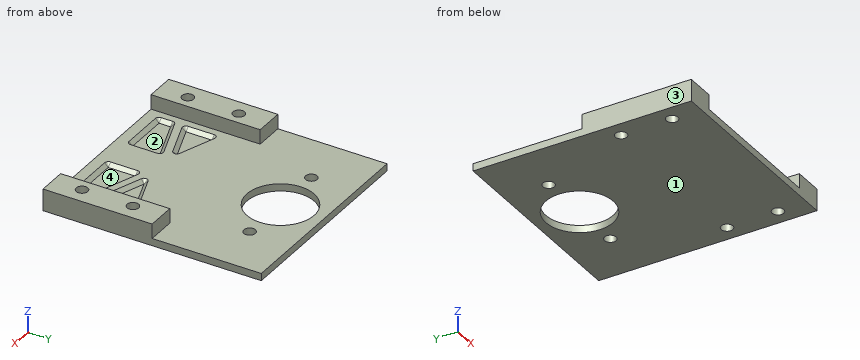
from build123d import *

# Parameters (mm, degrees)
SKIZZE1_W                       = 57
SKIZZE1_H                       = 60
GRUNDPLATTE_DEPTH               = 2
SKIZZE2_R                       = 9.25
SKIZZE2_R_2                     = 1.6
AUSSCHNITT_ROLLE_DEPTH          = 67.454871906
SKIZZE4_W                       = 8
SKIZZE4_H                       = 30
AUFSATZ_GETRIEBE_DEPTH          = 4
BOHRUNGEN_START                 = 4
SKIZZE3_R                       = 1.6
BOHRUNGEN_GETRIEBE_DEPTH        = 71.54509749
SCHNITT_LINEAR_AUSTRAGEN3_DEPTH = 1
VERRUNDUNG1_R                   = 1
FASE1_SIZE                      = 1


with BuildPart() as part:
    # Skizze1 → Grundplatte (new body)
    with BuildSketch(Plane.XY):
        with Locations((0, 30)):
            Rectangle(SKIZZE1_W, SKIZZE1_H)
    extrude(amount=GRUNDPLATTE_DEPTH)

    # Skizze2 → Ausschnitt_Rolle (cut, through all)
    with BuildSketch(Plane.XY.offset(2)):
        with Locations((0, 48)):
            Circle(SKIZZE2_R)
        with Locations((-14, 48)):
            Circle(SKIZZE2_R_2)
        with Locations(Location((14, 48, 0), (0, 0, 180))):
            Circle(SKIZZE2_R_2)
    extrude(amount=-AUSSCHNITT_ROLLE_DEPTH, mode=Mode.SUBTRACT)

    # Skizze4 → Aufsatz Getriebe (add)
    with BuildSketch(Plane.XY.offset(2)):
        with Locations((24.5, 15)):
            Rectangle(SKIZZE4_W, SKIZZE4_H)
        with Locations((-24.5, 15)):
            Rectangle(SKIZZE4_W, SKIZZE4_H)
    extrude(amount=AUFSATZ_GETRIEBE_DEPTH)

    # Skizze3 → Bohrungen Getriebe (cut, through all)
    with BuildSketch(Plane.XY.offset(2).offset(BOHRUNGEN_START)):
        with Locations(Location((-24, 22, 0), (0, 0, 180))):
            Circle(SKIZZE3_R)
        with Locations(Location((-24, 8, 0), (0, 0, 180))):
            Circle(SKIZZE3_R)
        with Locations(Location((24, 8, 0), (0, 0, 180))):
            Circle(SKIZZE3_R)
        with Locations(Location((24, 22, 0), (0, 0, 180))):
            Circle(SKIZZE3_R)
    extrude(amount=-BOHRUNGEN_GETRIEBE_DEPTH, mode=Mode.SUBTRACT)

    # Skizze5 → Schnitt-Linear austragen3 (cut)
    with BuildSketch(Plane.XY.offset(2)):
        Polygon((-18.5, 20), (-18.5, 10), (-4.5, 15), align=None)
        Polygon((-18.5, 7.876275893), (-18.5, 3), (-4.5, 3), (-4.5, 12.876275893), align=None)
        Polygon((4.5, 12.876275893), (18.5, 7.876275893), (18.5, 3), (4.5, 3), align=None)
        Polygon((4.5, 15), (18.5, 20), (18.5, 10), align=None)
    extrude(amount=-SCHNITT_LINEAR_AUSTRAGEN3_DEPTH, mode=Mode.SUBTRACT)

    # Verrundung1
    verrundung1_edges = [part.edges().sort_by_distance(p)[0] for p in [
        (-18.5, 3, 1.5),
        (-4.5, 3, 1.5),
        (-4.5, 12.876275893, 1.5),
        (-18.5, 7.876275893, 1.5),
        (18.5, 20, 1.5),
        (4.5, 15, 1.5),
        (18.5, 10, 1.5),
        (18.5, 3, 1.5),
        (18.5, 7.876275893, 1.5),
        (4.5, 12.876275893, 1.5),
        (4.5, 3, 1.5),
        (-18.5, 10, 1.5),
        (-4.5, 15, 1.5),
        (-18.5, 20, 1.5),
    ]]
    fillet(verrundung1_edges, radius=VERRUNDUNG1_R)

    # Fase1
    fase1_edges = [part.edges().sort_by_distance(p)[0] for p in [
        (4.923951563, 12.274686543, 1),
        (11.836336397, 10.256155751, 1),
        (18.31741556, 7.747605134, 1),
        (18.5, 5.585778349, 1),
        (18.207106781, 3.292893219, 1),
        (11.5, 3, 1),
        (4.792893219, 3.292893219, 1),
        (4.5, 7.728635491, 1),
        (18.076048437, 10.60158935, 1),
        (12.150270478, 12.267760544, 1),
        (6.473213749, 15, 1),
        (12.150270478, 17.732239456, 1),
        (18.076048437, 19.39841065, 1),
        (18.5, 15, 1),
        (-18.207106781, 3.292893219, 1),
        (-18.5, 5.585778349, 1),
        (-18.31741556, 7.747605134, 1),
        (-11.836336397, 10.256155751, 1),
        (-4.923951563, 12.274686543, 1),
        (-4.5, 7.728635491, 1),
        (-4.792893219, 3.292893219, 1),
        (-11.5, 3, 1),
        (-18.076048437, 10.60158935, 1),
        (-18.5, 15, 1),
        (-18.076048437, 19.39841065, 1),
        (-12.150270478, 17.732239456, 1),
        (-6.473213749, 15, 1),
        (-12.150270478, 12.267760544, 1),
    ]]
    chamfer(fase1_edges, length=FASE1_SIZE - 0.0001)  # a hair under: the kernel refuses the full size


solid = part.part
Verification items for the finished model (mm, model axes). Face numbers are marked on the shaded views. Round coordinates to 2 decimals unless told otherwise and drop trailing zeros. Loops run counter-clockwise (first coordinate to the right, second up) from the corner with the lowest first, then second, coordinate; pieces in that order, holes last. Notation, with made-up numbers: (-33, 23) - (25, 23) arc R18 ccw to (25, 55) - close; hole circle Ø3 at (0, -6.75). An arc over 180 degrees is marked (long way). Use a Markdown table: item, result. Add a question column.
1. Section check A-A, the plane y = 22. Record the boundary of the cut face in (x, z), plus the area to 3 significant figures.
2. Section check B-B, the plane z = 4. Record the boundary of the cut face in (x, y).
3. Thickness scan on probe 1 along Y at (x, z) = (-24, 4.55); probe 2 along X at (y, z) = (8, 3.85); probe 3 along Y at (x, z) = (0, 0.6). Record the ranges inside material, lowest first. Write a range as [from, to].
4. Release check for a two-part mould opening along X. For the marked faces 1, 2, 3 and 4 record: released by +X, released by -X, zero draft, split by the parting line, or undercut.
5. Gauge pin test, flat ends, axial feed: pin 1 (3.5 mm diameter, centred on x = 13, y = 16, fed in from +Z); pin 2 (24 mm diameter, centred on x = 0, y = 48, fed in from -Z); pin 3 (2 mm diameter, centred on x = 25, z = 5, fed in from +Y); pin 4 (5 mm diameter, centred on x = -14, y = 48, fed in from +Z). Record the tip position at first contact, or that the pin passes through.
6. Section check C-C, the plane x = 0. Record the boundary of the cut face in (y, z).
7. Section check D-D, the plane x = -24. Record the boundary of the cut face in (y, z), plus the area to 3 significant figures.
Checks:
| question | item | result |
|---|---|---|
| 1 | outline | (-28.5, 0) - (-25.6, 0) - (-25.6, 6) - (-28.5, 6) - close; (-22.4, 0) - (22.4, 0) - (22.4, 6) - (20.5, 6) - (20.5, 2) - (-20.5, 2) - (-20.5, 6) - (-22.4, 6) - close; (25.6, 0) - (28.5, 0) - (28.5, 6) - (25.6, 6) - close |
| 1 | area | 140 mm^2 |
| 2 | outline | (-28.5, 0) - (-20.5, 0) - (-20.5, 30) - (-28.5, 30) - close; (20.5, 0) - (28.5, 0) - (28.5, 30) - (20.5, 30) - close; hole circle Ø3.2 at (-24, 8); hole circle Ø3.2 at (-24, 22); hole circle Ø3.2 at (24, 8); hole circle Ø3.2 at (24, 22) |
| 3 | probe 1 | y = [0, 6.4], [9.6, 20.4], [23.6, 30] |
| 3 | probe 2 | x = [-28.5, -25.6], [-22.4, -20.5], [20.5, 22.4], [25.6, 28.5] |
| 3 | probe 3 | y = [0, 38.75], [57.25, 60] |
| 4 | face 1 | zero draft |
| 4 | face 2 | undercut |
| 4 | face 3 | released by -X |
| 4 | face 4 | undercut |
| 5 | pin 1 | stops at z = 1.83 |
| 5 | pin 2 | stops at z = 0 |
| 5 | pin 3 | stops at y = 30 |
| 5 | pin 4 | stops at z = 2 |
| 6 | outline | (0, 0) - (38.75, 0) - (38.75, 2) - (0, 2) - close; (57.25, 0) - (60, 0) - (60, 2) - (57.25, 2) - close |
| 7 | outline | (0, 0) - (6.4, 0) - (6.4, 6) - (0, 6) - close; (9.6, 0) - (20.4, 0) - (20.4, 6) - (9.6, 6) - close; (23.6, 0) - (60, 0) - (60, 2) - (30, 2) - (30, 6) - (23.6, 6) - close |
| 7 | area | 202 mm^2 |
